```python
from build123d import *

# Parameters (mm, degrees)
F1_DEPTH = 40
F3_D     = 5
F5_DEPTH = 20
F6_R     = 3


with BuildPart() as f1:
    # F0 (on Front) → F1 (new body)
    with BuildSketch(Plane.XZ):
        Polygon((0, 40), (0, 0), (40, 0), (40, 2), (2, 2), (2, 40), align=None)
    extrude(amount=F1_DEPTH)

    # F3 (through all)
    with Locations(Plane(origin=(0, 0, 0), x_dir=(0, -1, 0), z_dir=(-1, 0, 0))):
        with Locations((5, 5), (5, 35), (35, 5), (35, 35)):
            Hole(F3_D / 2)

    # F4 (on face) → F5 (cut)
    with BuildSketch(Plane(origin=(0, 0, 0), x_dir=(0, -1, 0), z_dir=(-1, 0, 0))):
        with BuildLine():
            Line((18.5, 28.506096), (18.5, 31.506096))
            ThreePointArc((18.5, 31.506096), (20, 8.396542), (21.5, 31.506096))
            Line((21.5, 31.506096), (21.5, 28.506096))
            Line((21.5, 28.506096), (20, 28.506096))
            Line((20, 28.506096), (18.5, 28.506096))
        make_face()
    extrude(amount=-F5_DEPTH, mode=Mode.SUBTRACT)

    # F6
    f6_edges = [f1.edges().sort_by_distance(p)[0] for p in [
        (1, -40, 40),
        (1, 0, 40),
        (40, -40, 1),
        (40, 0, 1),
    ]]
    fillet(f6_edges, radius=F6_R)


solid = f1.part
```
Geometry: final body of the model. Coordinates: model frame, mm. A direction names the side the tool comes from. Give positions to 0.01 mm unless a question says otherwise; leave off trailing zeros. Loops run counter-clockwise (first coordinate to the right, second up) from the corner with the lowest first, then second, coordinate; pieces in that order, holes last. Notation, with made-up numbers: (48.25, 23) -> (105.25, 23) arc R26 cw to (105.25, 55) -> close; hole circle Ø6 at (22, 21.25). An arc over 180 degrees is marked (long way). Use CSV: the item, a comma, the result in double quotes.
(1) Cut plane B-B (z = 20). Output: boundary loops of the cut face in (x, y).
From the geometry:
outline,"(0, -40) -> (2, -40) -> (2, -31.6) -> (0, -31.6) -> close; (0, -8.4) -> (2, -8.4) -> (2, 0) -> (0, 0) -> close"
(2) Cut plane C-C (z = 5). Output: boundary loops of the cut face in (x, y).
From the geometry:
outline,"(0, -40) -> (2, -40) -> (2, -37.5) -> (0, -37.5) -> close; (0, -32.5) -> (2, -32.5) -> (2, -7.5) -> (0, -7.5) -> close; (0, -2.5) -> (2, -2.5) -> (2, 0) -> (0, 0) -> close"
(3) First-contact query: P1, Ø18.5, axis at y = -20, z = 20, coming from the +X side; P2, Ø1.5, axis at x = 16, y = -4.5, coming from the +Z side; P3, Ø3, axis at y = -5, z = 35, coming from the +X side. Flat tips, straight axial feed; report the tip coordinate or a pass-through.
From the geometry:
P1,"x = 2"
P2,"z = 2"
P3,"through"
(4) Pull-direction query (Z, two-part tool) for faces 1 (the face through (40, -20, 1)), 2 (the face through (1.01, -32.69, 34.04)), 3 (the face through (1, -20, 40)); classes: released by +Z, released by -Z, zero draft, split by the parting line, or undercut.
From the geometry:
face 1,"zero draft"
face 2,"undercut"
face 3,"released by +Z"
(5) Cut plane A-A (y = -20). Output: boundary loops of the cut face in (x, z).
From the geometry:
outline,"(0, 0) -> (40, 0) -> (40, 2) -> (2, 2) -> (2, 8.4) -> (0, 8.4) -> close; (0, 28.51) -> (2, 28.51) -> (2, 40) -> (0, 40) -> close"
(6) Access query for faces 4 (the face through (0, -20, 29)), 5 (the face through (21, -20, 2)), 6 (the face through (1, -18.5, 30)). Directions: +Z, -Z, +X, -X, +Y, -Y. A direction counts if a zero-diameter tool reaches every point of the face in a straight line with its end or side. Return the directions, or none.
From the geometry:
face 4,"+Z, -Z, -X, +Y, -Y"
face 5,"+Z, +X, +Y, -Y"
face 6,"+X, -X"
(7) Ray query, line 1 along Z through (x, y) = (0.8, -35); line 2 along Z through (x, y) = (0.4, -20); line 3 along Y through (x, z) = (1.1, 20). Return the intervals inside material, ascending. Write a range as [from, to].
From the geometry:
line 1,"[0, 2.5], [7.5, 32.5], [37.5, 40]"
line 2,"[0, 8.4], [28.51, 40]"
line 3,"[-40, -31.6], [-8.4, 0]"
(8) Cut plane D-D (y = -35). Output: boundary loops of the cut face in (x, z).
From the geometry:
outline,"(0, 0) -> (40, 0) -> (40, 2) -> (2, 2) -> (2, 2.5) -> (0, 2.5) -> close; (0, 7.5) -> (2, 7.5) -> (2, 32.5) -> (0, 32.5) -> close; (0, 37.5) -> (2, 37.5) -> (2, 40) -> (0, 40) -> close"
